CAD build for the part. Positions are in the model's coordinates, mm. A direction names the side the tool comes from. Coordinates: 2 decimals unless noted, no trailing zeros. Loops run counter-clockwise (first coordinate to the right, second up) from the corner with the lowest first, then second, coordinate; pieces in that order, holes last. Notation, with made-up numbers: (27.25, 39.25) -> (48.25, 39.25) arc R25 ccw to (48.25, 62.25) -> close; hole circle Ø2 at (-39, -17.5). An arc over 180 degrees is marked (long way). Write each question's results on one line, items separated by ' | '.
```python
from build123d import *

# Parameters (mm, degrees)
SKETCH_5_R               = 2.5
EXTRUDE_3_DEPTH          = 15
SKETCH_1_R               = 35
SKETCH_1_R_2             = 5
EXTRUDE_4_DEPTH          = 3
CUT_EXTRUDE_1_DEPTH      = 54.200093985
CUT_EXTRUDE_1_DEPTH_BACK = 54.200093985
SKETCH_4_W               = 25
SKETCH_4_H               = 12


with BuildPart() as part:
    # 스케치5 → 보스-돌출3 (new, symmetric)
    with BuildSketch(Plane(origin=(0, 0, 0), x_dir=(1, 0, 0), z_dir=(0, 1, 0))):
        with BuildLine():
            Line((-10, 0), (10, 0))
            Line((10, 0), (5.262640911, 15.598314937))
            ThreePointArc((5.262640911, 15.598314937), (0, 19.5), (-5.262640911, 15.598314937))
            Line((-5.262640911, 15.598314937), (-10, 0))
        make_face()
        with Locations(Location((0, 14, 0), (0, 0, 270))):
            Circle(SKETCH_5_R, mode=Mode.SUBTRACT)
    extrude(amount=EXTRUDE_3_DEPTH, both=True)

    # 스케치1 → 보스-돌출4 (add)
    with BuildSketch(Plane.XY):
        Circle(SKETCH_1_R)
        with BuildLine():
            ThreePointArc((32.5, 0), (30, -2.5), (27.5, 0))
            ThreePointArc((27.5, 0), (19.445436483, 19.445436483), (0, 27.5))
            ThreePointArc((0, 27.5), (-2.5, 30), (0, 32.5))
            ThreePointArc((0, 32.5), (22.980970389, 22.980970389), (32.5, 0))
        make_face(mode=Mode.SUBTRACT)
        with BuildLine():
            ThreePointArc((0, -27.5), (2.5, -30), (0, -32.5))
            ThreePointArc((0, -32.5), (-22.980970405, -22.980970372), (-32.5, 4.6e-08))
            ThreePointArc((-32.5, 4.6e-08), (-29.999999977, 2.5), (-27.5, 0))
            ThreePointArc((-27.5, 0), (-19.445436483, -19.445436483), (0, -27.5))
        make_face(mode=Mode.SUBTRACT)
        Circle(SKETCH_1_R_2, mode=Mode.SUBTRACT)
    extrude(amount=EXTRUDE_4_DEPTH)

    # 스케치4 → 컷-돌출1 (cut, two sides: drawn at the far end of the back side and taken through both)
    with BuildSketch(Plane(origin=(0, 0, 0), x_dir=(0, 0, -1), z_dir=(1, 0, 0)).offset(-CUT_EXTRUDE_1_DEPTH_BACK)):
        with Locations((12.5, 0)):
            Rectangle(SKETCH_4_W, SKETCH_4_H)
    extrude(amount=CUT_EXTRUDE_1_DEPTH + CUT_EXTRUDE_1_DEPTH_BACK, mode=Mode.SUBTRACT)


solid = part.part
```
Q1. Which spindle directions (+Z, -Z, +X, -X, +Y, -Y) get a long thin tool onto all of the face, cutting with end or side? Do faces 4 (the cylindrical face through (19.66, 19.23, 1.48)), 5 (the flat face through (0, -15, -8)), 6 (the flat face through (0, 6, -7)). Say none if no direction does.
Results are:
face 4: +Z, -Z | face 5: -Z, +X, -X, -Y | face 6: -Z, +X, -X
Q2. Cut at D-D on z = 1.75. Write the cut outline in (x, y).
Results are:
outline: circle Ø70 at (0, 0); hole (-32.5, 0) arc R32.5 ccw to (0, -32.5) arc R2.5 ccw to (0, -27.5) arc R27.5 cw to (-27.5, 0) arc R2.5 ccw to start; hole circle Ø10 at (0, 0); hole (0, 27.5) arc R27.5 cw to (27.5, 0) arc R2.5 ccw to (32.5, 0) arc R32.5 ccw to (0, 32.5) arc R2.5 ccw to start
Q3. Wall check: L1, parallel to Y at x = -2, z = -11.5; L2, parallel to Z at x = 6.5, y = 32; L3, parallel to X at y = 13.25, z = -14. Give the ranges that are in metal, low to high. Write a range as from..to.
Results are:
L1: -15..-6, 6..15 | L2: 0..3 | L3: -5.75..-2.5, 2.5..5.75
Q4. Pull direction Y, two halves, no side cores. Call faces 1 (the cylindrical face through (-22.73, -23.23, 1.48)), 2 (the cylindrical face through (-28, -21, 1)), 3 (the flat face through (0, -7, 3)): +Y half, -Y half, draft (parallel to the pull), parting line (faces both ways), or undercut.
Results are:
face 1: undercut | face 2: parting line | face 3: draft
Q5. Cut at C-C on x = -30. Write the cut outline in (y, z).
Results are:
outline: (-18.03, 0) -> (-12.5, 0) -> (-12.5, 3) -> (-18.03, 3) -> close; (2.5, 0) -> (18.03, 0) -> (18.03, 3) -> (2.5, 3) -> close
Q6. Drop flat-ended pins along their axis: pin 1 (6 mm diameter, centred on x = 18, y = -17.5, fed in from -Z); pin 2 (10 mm diameter, centred on x = 9.5, y = -11.5, fed in from -Z); pin 3 (6 mm diameter, centred on x = -3, z = -12.5, fed in from +Y). Give the stop position or say it passes through.
Results are:
pin 1: z = 0 | pin 2: z = -17.16 | pin 3: y = 15
Q7. Cut at B-B on z = -2.5. Write the cut outline in (x, y), and give its area (3 significant figures).
Results are:
outline: (-9.24, -15) -> (9.24, -15) -> (9.24, -6) -> (-9.24, -6) -> close; (-9.24, 6) -> (9.24, 6) -> (9.24, 15) -> (-9.24, 15) -> close | area: 333 mm^2
Q8. Cut at A-A on y = 4. Write the cut outline in (x, z), and give its area (3 significant figures).
Results are:
outline: (-34.77, 0) -> (-3, 0) -> (-3, 3) -> (-34.77, 3) -> close; (3, 0) -> (27.21, 0) -> (27.21, 3) -> (3, 3) -> close; (32.25, 0) -> (34.77, 0) -> (34.77, 3) -> (32.25, 3) -> close | area: 175 mm^2
